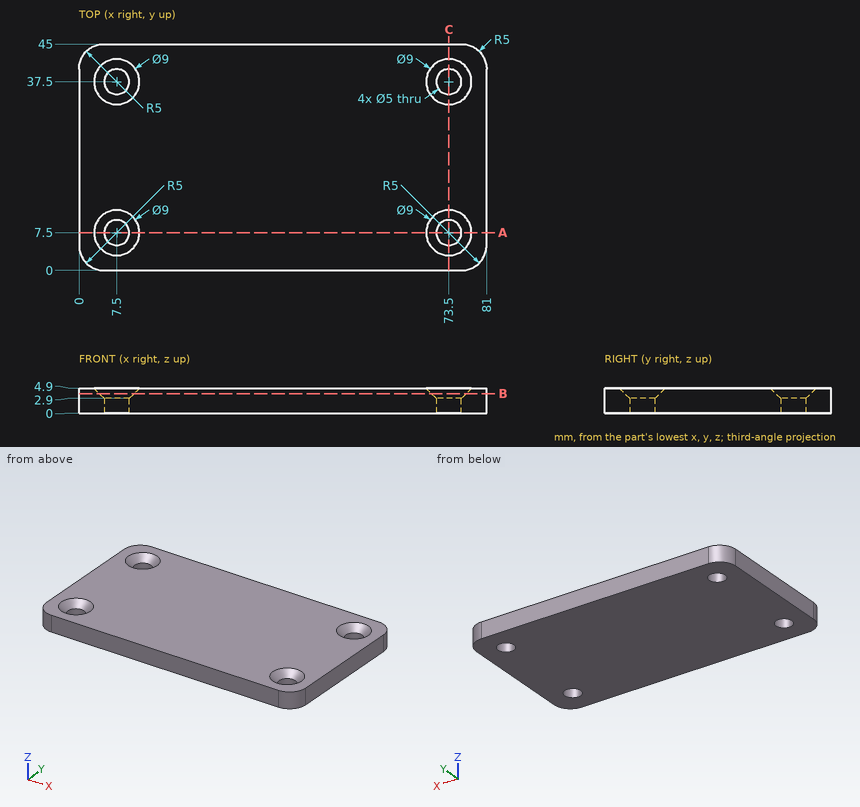
Job drawing, mm, ordinate dimensions from the low corner. One solid piece. Round coordinates to 2 decimals unless told otherwise and drop trailing zeros. Loops run counter-clockwise (first coordinate to the right, second up) from the corner with the lowest first, then second, coordinate; pieces in that order, holes last.
Item 1: Cut at A-A, the plane y = 7.5. Give the cut face in (x, z), then the cut area to 3 significant figures.
Item 2: Cut at C-C, the plane x = 73.5. Give the cut face in (y, z).
Item 3: Cut at B-B, the plane z = 3.85. Give the cut face in (x, y).
Item 4: Drill centre lines: line 1 (Y direction, x = 73.5, z = 1.5); line 2 (X direction, y = 35.5, z = 2); line 3 (X direction, y = 5.5, z = 4.7). Where is each one in solid material? Low to high.
A:
1. outline: (0, 0) - (5, 0) - (5, 2.9) - (3, 4.9) - (0, 4.9) - close; (10, 0) - (71, 0) - (71, 2.9) - (69, 4.9) - (12, 4.9) - (10, 2.9) - close; (76, 0) - (81, 0) - (81, 4.9) - (78, 4.9) - (76, 2.9) - close
1. area: 340 mm2
2. outline: (0, 0) - (5, 0) - (5, 2.9) - (3, 4.9) - (0, 4.9) - close; (10, 0) - (35, 0) - (35, 2.9) - (33, 4.9) - (12, 4.9) - (10, 2.9) - close; (40, 0) - (45, 0) - (45, 4.9) - (42, 4.9) - (40, 2.9) - close
3. outline: (0, 5) arc R5 ccw to (5, 0) - (76, 0) arc R5 ccw to (81, 5) - (81, 40) arc R5 ccw to (76, 45) - (5, 45) arc R5 ccw to (0, 40) - close; hole circle Ø6.9 at (7.5, 7.5); hole circle Ø6.9 at (7.5, 37.5); hole circle Ø6.9 at (73.5, 7.5); hole circle Ø6.9 at (73.5, 37.5)
4. line 1: y = 0 to 5, 10 to 35, 40 to 45
4. line 2: x = 0 to 6, 9 to 72, 75 to 81
4. line 3: x = 0 to 3.69, 11.31 to 69.69, 77.31 to 81
